Autodesk Inventor part; units mm, degrees
ref_plane "YZ Plane" through (0, 0, 0) normal (1, 0, 0) x (0, 1, 0)
ref_plane "XZ Plane" through (0, 0, 0) normal (0, 1, 0) x (-1, 0, 0)
ref_plane "XY Plane" through (0, 0, 0) normal (0, 0, 1) x (1, 0, 0)
sketch "Sketch1" plane through (0, 0, 0) normal (1, 0, 0) x (0, 1, 0)
  line L0 (0, 0) -> (0, 15.4021) construction
  line L1 (-80, 0) -> (0, 0) construction
  line L2 (-10, 16) -> (-10, 44) construction
  line L3 (-10, 56) -> (-10, 0)
  line L4 (-10, 0) -> (-80, 0)
  line L5 (-80, 0) -> (-80, 6)
  line L6 (-80, 6) -> (-30, 56)
  line L7 (-30, 56) -> (-10, 56)
  point P0 (-10, 28)
  dimension "d0" = 6
  dimension "d1" = 70
  dimension "d2" = 56
  dimension "d3" = 20
extrude "Extrusion1" add sketch "Sketch1" along normal mid plane 25
sketch "Sketch2" plane through (-12.5, -10, 56) normal (0, 1, 0) x (1, 0, 0)
  circle A0 centre (12.5, 12) radius 4.1 construction
  circle A1 centre (12.5, 30) radius 4.1 construction
  point P0 (12.5, 56)
hole "Hole1" at (0, -10, 44) at (0, -10, 26) direction (0, -1, 0) diameter 8.2 depth 16
sketch "Sketch3" plane through (-12.5, -80, 0) normal (0, -1, 0) x (1, 0, 0)
  circle A0 centre (12.5, 44) radius 4.1 construction
  circle A1 centre (12.5, 26) radius 4.1 construction
  point P0 (12.5, 0)
hole "Hole2" at (0, -80, 44) at (0, -80, 26) direction (0, 1, 0) diameter 14 depth 54
sketch "Sketch4" plane through (0, 0, 0) normal (0, 0, 1) x (1, 0, 0)
  line L0 (-30.5, -10) -> (30.5, -10)
  line L1 (30.5, -10) -> (30.5, -30)
  line L2 (30.5, -80) -> (-30.5, -80)
  line L3 (-30.5, -80) -> (-30.5, -60)
  line L4 (0, 0) -> (0, -133.7428) construction
  line L5 (-30.5, -30) -> (-12.5, -30) construction
  line L6 (-12.5, -30) -> (-12.5, -60) construction
  line L7 (-12.5, -10) -> (-12.5, -80) construction
  line L8 (-30.5, -60) -> (-12.5, -60) construction
  line L9 (30.5, -30) -> (12.5, -30) construction
  line L10 (12.5, -80) -> (12.5, -10) construction
  line L11 (12.5, -60) -> (30.5, -60) construction
  line L12 (12.5, -30) -> (12.5, -60) construction
  line L13 (-30.5, -60) -> (-30.5, -30)
  line L14 (30.5, -30) -> (30.5, -60)
  line L15 (30.5, -60) -> (30.5, -80)
  line L16 (-30.5, -30) -> (-30.5, -10)
  dimension "d20" = 30.5
  dimension "d36" = 20
  dimension "d37" = 20
extrude "Extrusion2" add sketch "Sketch4" along normal blind 6
sketch "Sketch5" plane through (0, 0, 6) normal (0, 0, 1) x (1, 0, 0)
  line L0 (-30.5, -10) -> (30.5, -10) construction
  line L1 (20.5, -10) -> (20.5, -80) construction
  line L2 (30.5, -80) -> (-30.5, -80) construction
  line L3 (30.5, -80) -> (30.5, -10) construction
  line L4 (0, 0) -> (0, -101.1083) construction
  line L5 (12.5, -30) -> (12.5, -80) construction
  line L6 (12.5, -80) -> (30.5, -80)
  point P0 (20.5, -20)
  point P1 (20.5, -70)
  point P2 (-20.5, -20)
  point P3 (-20.5, -70)
  point P4 (20.5, -45)
  point P5 (-20.5, -45)
  dimension "d24" = 10
  dimension "d35" = 50
  dimension "d50" = 25
  dimension "d53" = 10
hole "Hole3" at (-20.5, -70, 6) at (-20.5, -20, 6) at (20.5, -20, 6) at (20.5, -70, 6) at (-20.5, -45, 6) at (20.5, -45, 6) direction (0, 0, -1) diameter 6.2 end through all
fillet "Fillet1" radius 3 4 edges at (-30.5, -80, 3) (30.5, -80, 3) (30.5, -10, 3) (-30.5, -10, 3)
fillet "Fillet2" radius 3 2 edges at (-12.5, -20, 56) (12.5, -20, 56)
properties part number "LoadCell_NewBase" material "Aluminum 7075"
Part model, mm, in its own coordinate system. A direction names the side the tool comes from. Round coordinates to 2 decimals unless told otherwise and drop trailing zeros. Loops run counter-clockwise (first coordinate to the right, second up) from the corner with the lowest first, then second, coordinate; pieces in that order, holes last. Notation, with made-up numbers: (-34, 63.25) - (-10, 63.25) arc R6 cw to (-10, 71.25) - close; hole circle Ø2 at (33.25, 77). An arc over 180 degrees is marked (long way). Answer as a JSON object with one key per item and string values.
Item 1: Band-saw the part on B-B on y = -70. List the corners of the cut face in (x, z), plus the area to 3 significant figures.
Output:
{"outline": "(-30.5, 0) - (-23.6, 0) - (-23.6, 6) - (-30.5, 6) - close; (-17.4, 0) - (17.4, 0) - (17.4, 6) - (12.5, 6) - (12.5, 16) - (-12.5, 16) - (-12.5, 6) - (-17.4, 6) - close; (23.6, 0) - (30.5, 0) - (30.5, 6) - (23.6, 6) - close", "area": "542 mm2"}
Item 2: Band-saw the part on D-D on x = -20.5. List the corners of the cut face in (y, z), plus the area to 3 significant figures.
Output:
{"outline": "(-80, 0) - (-73.1, 0) - (-73.1, 6) - (-80, 6) - close; (-66.9, 0) - (-48.1, 0) - (-48.1, 6) - (-66.9, 6) - close; (-41.9, 0) - (-23.1, 0) - (-23.1, 6) - (-41.9, 6) - close; (-16.9, 0) - (-10, 0) - (-10, 6) - (-16.9, 6) - close", "area": "308 mm2"}
Item 3: Pin check, flat tips, straight feed: pin 1 (5.5 mm diameter, centred on x = -23.5, y = -39.5, fed in from +Z); pin 2 (23.5 mm diameter, centred on y = -48.5, z = 19.5, fed in from +X); pin 3 (5 mm diameter, centred on x = -20.5, y = -45, fed in from -Z); pin 4 (23.5 mm diameter, centred on y = -42.5, z = 31, fed in from -X). Stop position of each tip, or through.
Output:
{"pin 1": "z = 6", "pin 2": "x = 12.5", "pin 3": "through", "pin 4": "x = -12.5"}
Item 4: Wall check: L1, parallel to X at y = -70, z = 4.25; L2, parallel to Y at x = 20.5, z = 4.2; L3, parallel to X at y = -21.5, z = 44. Give the ranges that are in metal, low to high.
Output:
{"L1": "-30.5 to -23.6, -17.4 to 17.4, 23.6 to 30.5", "L2": "-80 to -73.1, -66.9 to -48.1, -41.9 to -23.1, -16.9 to -10", "L3": "-12.5 to -4.1, 4.1 to 12.5"}
Item 5: Tool access for faces 1 (the face through (-24, -45, 6)), 2 (the face through (-6, -55, 31)), 3 (the face through (25, -45, 6)), 4 (the face through (3.01, -26, 40.99)), 5 (the face through (29.64, -10.9, 3.04)): list every direction of +Z, -Z, +X, -X, +Y, -Y with a clear straight run to the whole face (end or side of a thin tool).
Output:
{"face 1": "+Z, -X, +Y, -Y", "face 2": "+Z, +X, -X, -Y", "face 3": "+Z, +X, +Y, -Y", "face 4": "-Y", "face 5": "+Z, -Z, +X, +Y"}
Item 6: Band-saw the part on A-A on x = 0. List the corners of the cut face in (y, z), plus the area to 3 significant figures.
Output:
{"outline": "(-80, 0) - (-10, 0) - (-10, 21.9) - (-26, 21.9) - (-26, 19) - (-67, 19) - (-80, 6) - close; (-53, 33) - (-26, 33) - (-26, 30.1) - (-10, 30.1) - (-10, 39.9) - (-26, 39.9) - (-26, 37) - (-49, 37) - close; (-35, 51) - (-26, 51) - (-26, 48.1) - (-10, 48.1) - (-10, 56) - (-30, 56) - close", "area": "1,710 mm2"}
Item 7: Band-saw the part on C-C on z = 26. List the corners of the cut face in (x, y), plus the area to 3 significant figures.
Output:
{"outline": "(-12.5, -60) - (-7, -60) - (-7, -26) - (-4.1, -26) - (-4.1, -10) - (-12.5, -10) - close; (4.1, -26) - (7, -26) - (7, -60) - (12.5, -60) - (12.5, -10) - (4.1, -10) - close", "area": "643 mm2"}
Item 8: Pull direction X, two halves, no side cores. Call faces 6 (the face through (-12.5, -38, 25)), 7 (the face through (-18.614, -17.54, 2.958)), 8 (the face through (12.5, -38, 25)): pulls with the +X half, pulls with the -X half, needs draft (parallel to the pull), parting line crosses it, or undercut.
Output:
{"face 6": "pulls with the -X half", "face 7": "undercut", "face 8": "pulls with the +X half"}
